The listing builds one solid part. Answer for the finished solid, in the listing's coordinates (mm). Give positions to 0.01 mm unless a question says otherwise; leave off trailing zeros. Loops run counter-clockwise (first coordinate to the right, second up) from the corner with the lowest first, then second, coordinate; pieces in that order, holes last. Notation, with made-up numbers: (58.5, -28) - (80.5, -28) arc R21 ccw to (80.5, 3) - close; hole circle Ø4 at (74.25, 24). An arc over 180 degrees is marked (long way). Write each question's results on one line, items separated by ' | '.
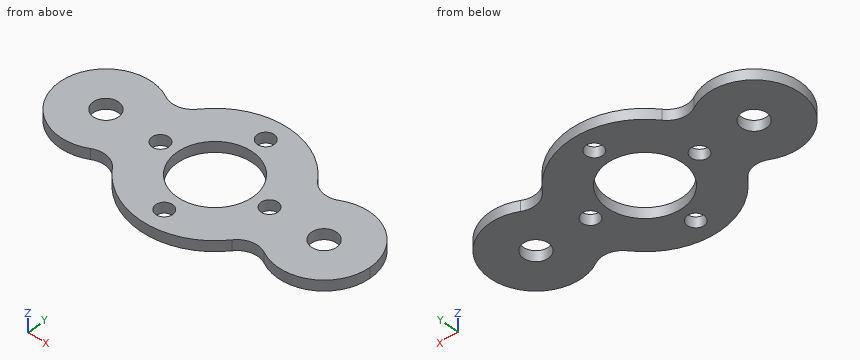
from build123d import *

# Parameters (mm, degrees)
F0_R     = 3
F0_R_2   = 2
F0_R_3   = 9
F1_DEPTH = 2.5
F2_R     = 5


with BuildPart() as f1:
    # F0 (on Top) → F1 (new body)
    with BuildSketch(Plane.XY):
        with BuildLine():
            ThreePointArc((16.9038461538, -6.1854656419), (17.7238431325, -3.140920982), (18, 0))
            ThreePointArc((18, 0), (17.7238431325, 3.140920982), (16.9038461538, 6.1854656419))
            ThreePointArc((16.9038461538, 6.1854656419), (15.4867299971, 3.2359162298), (15, 0))
            ThreePointArc((15, 0), (15.4867299971, -3.2359162298), (16.9038461538, -6.1854656419))
        make_face()
        with BuildLine():
            ThreePointArc((16.9038461538, 6.1854656419), (17.7238431325, 3.140920982), (18, 0))
            ThreePointArc((18, 0), (17.7238431325, -3.140920982), (16.9038461538, -6.1854656419))
            ThreePointArc((16.9038461538, -6.1854656419), (29.2359162298, -10.5132700029), (37, 0))
            ThreePointArc((37, 0), (29.2359162298, 10.5132700029), (16.9038461538, 6.1854656419))
        make_face()
        with Locations((26, 0)):
            Circle(F0_R, mode=Mode.SUBTRACT)
        with BuildLine():
            ThreePointArc((15, 0), (15.4867299971, 3.2359162298), (16.9038461538, 6.1854656419))
            ThreePointArc((16.9038461538, 6.1854656419), (0, 18), (-16.9038461538, 6.1854656419))
            ThreePointArc((-16.9038461538, 6.1854656419), (-15.4867299971, 3.2359162298), (-15, 0))
            ThreePointArc((-15, 0), (-15.4867299971, -3.2359162298), (-16.9038461538, -6.1854656419))
            ThreePointArc((-16.9038461538, -6.1854656419), (0, -18), (16.9038461538, -6.1854656419))
            ThreePointArc((16.9038461538, -6.1854656419), (15.4867299971, -3.2359162298), (15, 0))
        make_face()
        with Locations((0, -13)):
            Circle(F0_R_2, mode=Mode.SUBTRACT)
        with BuildLine():
            ThreePointArc((-11, 0), (-13, -2), (-15, 0))
            ThreePointArc((-15, 0), (-13, 2), (-11, 0))
        make_face(mode=Mode.SUBTRACT)
        Circle(F0_R_3, mode=Mode.SUBTRACT)
        with Locations((13, 0)):
            Circle(F0_R_2, mode=Mode.SUBTRACT)
        with Locations((0, 13)):
            Circle(F0_R_2, mode=Mode.SUBTRACT)
        with BuildLine():
            ThreePointArc((-15, 0), (-15.4867299971, 3.2359162298), (-16.9038461538, 6.1854656419))
            ThreePointArc((-16.9038461538, 6.1854656419), (-18, 0), (-16.9038461538, -6.1854656419))
            ThreePointArc((-16.9038461538, -6.1854656419), (-15.4867299971, -3.2359162298), (-15, 0))
        make_face()
        with BuildLine():
            ThreePointArc((-16.9038461538, -6.1854656419), (-18, 0), (-16.9038461538, 6.1854656419))
            ThreePointArc((-16.9038461538, 6.1854656419), (-37, 0), (-16.9038461538, -6.1854656419))
        make_face()
        with Locations((-26, 0)):
            Circle(F0_R, mode=Mode.SUBTRACT)
    extrude(amount=F1_DEPTH)

    # F2
    f2_edges = [f1.edges().sort_by_distance(p)[0] for p in [
        (16.903846, 6.185466, 1.25),
        (-16.903846, 6.185466, 1.25),
        (16.903846, -6.185466, 1.25),
        (-16.903846, -6.185466, 1.25),
    ]]
    fillet(f2_edges, radius=F2_R)


solid = f1.part
Item 1: A cutting plane is placed at A-A, the plane x = 0. Determine the outline of the cut face in (y, z).
Values found:
outline: (-18, 0) - (-15, 0) - (-15, 2.5) - (-18, 2.5) - close; (-11, 0) - (-9, 0) - (-9, 2.5) - (-11, 2.5) - close; (9, 0) - (11, 0) - (11, 2.5) - (9, 2.5) - close; (15, 0) - (18, 0) - (18, 2.5) - (15, 2.5) - close
Item 2: Flat-ended cylindrical pins translate along their axes: P1, Ø2.5, axis at x = -13, y = 0, coming from the +Z side; P2, Ø1, axis at x = -10, z = 1, coming from the +Y side; P3, Ø1, axis at x = -4.5, z = 1, coming from the -Y side. Find the tip coordinate at first contact, or state that the pin passes through.
Values found:
P1: passes through | P2: stops at y = 15.29 | P3: stops at y = -17.55
Item 3: Find the intervals of material crossed by line 1 along Y through (x, z) = (-26, 1.9); line 2 along Y through (x, z) = (-13, 0.75); line 3 along X through (y, z) = (-14.5, 2.15), in increasing order. Write a range as [from, to].
Values found:
line 1: y = [-11, -3], [3, 11] | line 2: y = [-12.45, -2], [2, 12.45] | line 3: x = [-10.67, -1.32], [1.32, 10.67]
Item 4: A cutting plane is placed at C-C, the plane y = 13. Determine the outline of the cut face in (x, z).
Values found:
outline: (-12.45, 0) - (-2, 0) - (-2, 2.5) - (-12.45, 2.5) - close; (2, 0) - (12.45, 0) - (12.45, 2.5) - (2, 2.5) - close
Item 5: A cutting plane is placed at D-D, the plane z = 0.9. Count the separate pieces of the cut face and the enclosed holes in it, plus the area to 3 significant figures.
Values found:
separate pieces: 1 | enclosed holes: 7 | area: 1,390 mm²
Item 6: A cutting plane is placed at B-B, the plane x = 7.5. Determine the outline of the cut face in (y, z), plus the area to 3 significant figures.
Values found:
outline: (-16.36, 0) - (-4.97, 0) - (-4.97, 2.5) - (-16.36, 2.5) - close; (4.97, 0) - (16.36, 0) - (16.36, 2.5) - (4.97, 2.5) - close | area: 56.9 mm²
